Build history of the part. All positions in model axes, mm. A direction names the side the tool comes from. Coordinates: 2 decimals unless noted, no trailing zeros. Order: outer loops, then holes, each group sorted by start corner. A loop starts at its lowest first (then second) coordinate and runs counter-clockwise, first axis right, second up. Notation, with made-up numbers: M 85.5,-26 L 119.5,-26 A10 ccw 119.5,-22 Z; hole C 89.5,-15 d3. An arc over 180 degrees is marked long. Use a Markdown table: item, result. Add a question column.
from build123d import *

# Parameters (mm, degrees)
ESTRUSIONE_ESTRUSIONE1_DEPTH = 2
SCHIZZO2_W                   = 7
SCHIZZO2_H                   = 5
ESTRUSIONE_ESTRUSIONE2_DEPTH = 6.5
FORO_PER_VITE_M3_1_D         = 3.4
FORO_PER_VITE_M3_1_DEPTH     = 2
FORO_PER_VITE_M3_1_TIP       = 1.021463052
FORO_PER_VITE_M3_2_D         = 3.4
RACCORDO1_RADIUS             = 3.5
RACCORDO1_LENGTH             = 5
SMUSSO1_SIZE                 = 1
RACCORDO2_R                  = 1


with BuildPart() as part:
    # Schizzo1 → Estrusione-Estrusione1 (new body)
    with BuildSketch(Plane.XY):
        Polygon((5, 5), (5, 0), (14, 0), (14, -5), (5, -5), (-5, -5), (-5, 5), align=None)
    extrude(amount=ESTRUSIONE_ESTRUSIONE1_DEPTH)

    # Schizzo2 → Estrusione-Estrusione2 (add)
    with BuildSketch(Plane.XY.offset(2)):
        with Locations((10.5, -2.5)):
            Rectangle(SCHIZZO2_W, SCHIZZO2_H)
    extrude(amount=ESTRUSIONE_ESTRUSIONE2_DEPTH)

    # Foro per Vite M3-1
    with Locations(Plane.XY.offset(2)):
        with Locations((0, 0)):
            Hole(FORO_PER_VITE_M3_1_D / 2, depth=FORO_PER_VITE_M3_1_DEPTH)
            with Locations((0, 0, -(FORO_PER_VITE_M3_1_DEPTH + FORO_PER_VITE_M3_1_TIP / 2))):  # 118° drill point
                Cone(0, FORO_PER_VITE_M3_1_D / 2, FORO_PER_VITE_M3_1_TIP, mode=Mode.SUBTRACT)

    # Foro per Vite M3-2 (through all)
    with Locations(Plane(origin=(0, -5, 0), x_dir=(-1, 0, 0), z_dir=(0, -1, 0))):
        with Locations((-10.5, -5.25)):
            Hole(FORO_PER_VITE_M3_2_D / 2)

    # Raccordo1: full round fillet: the end face becomes a half cylinder, R = half its width
    raccordo1_face = Plane((10.5, -2.5, 8.5), x_dir=(0, 1, 0), z_dir=(0, 0, 1))  # on the end face: x along it, z out of the body
    raccordo1_slab = raccordo1_face.offset(-RACCORDO1_RADIUS / 2) * Box(RACCORDO1_LENGTH, 2 * RACCORDO1_RADIUS, RACCORDO1_RADIUS, mode=Mode.PRIVATE)  # the body's end, R deep
    raccordo1_round = Plane((10.5, -2.5, 5), x_dir=(0, 0, 1), z_dir=(0, 1, 0)) * Cylinder(RACCORDO1_RADIUS, RACCORDO1_LENGTH, mode=Mode.PRIVATE)  # its axis R under the face
    add(raccordo1_slab - raccordo1_round, mode=Mode.SUBTRACT)

    # Smusso1
    smusso1_edges = [part.edges().sort_by_distance(p)[0] for p in [
        (14, -2.5, 0),
    ]]
    chamfer(smusso1_edges, length=SMUSSO1_SIZE)

    # Raccordo2
    raccordo2_edges = [part.edges().sort_by_distance(p)[0] for p in [
        (14, -2.5, 1),
        (13, -2.5, 0),
    ]]
    fillet(raccordo2_edges, radius=RACCORDO2_R)


solid = part.part
(1) Drop flat-ended pins along their axis: P1, Ø3, axis at y = 1, z = 7, coming from the -X side; P2, Ø2.5, axis at x = 0, y = 0, coming from the +Z side; P3, Ø4, axis at x = 8, z = 3.5, coming from the +Y side; P4, Ø1, axis at y = 2, z = 1, coming from the +X side. Give the stop position or say it passes through.
(2) Slice it at B-B on x = 10.5. Give the cut face in (y, z).
(3) Drill centre lines: line 1 along Y through (x, z) = (0, 0.5); line 2 along Z through (x, y) = (3.25, -4); line 3 along X through (y, z) = (-1.25, 5.25). Where is each one in solid material? Low to high. Write a range as from..to.
(4) Slice it at D-D on x = 5.25. Give the cut face in (y, z), and give its area (3 significant figures).
(5) Slice it at A-A on y = -2.5. Give the cut face in (x, z).
(6) Which spindle directions (+Z, -Z, +X, -X, +Y, -Y) get a long thin tool onto all of the face, cutting with end or side? Do faces 4 (the cylindrical face through (10.4, -2.5, 8.5)), 5 (the flat face through (1, -2, 2)), 6 (the flat face through (5, 3, 1)). Say none if no direction does.
(7) Slice it at C-C on z = 5.25. Give the cut face in (x, y).
(8) Mould opens along X. For faces 1 (the flat face through (7, -3, 3)), 2 (the flat face through (0, 5, 1)), 3 (the cylindrical face through (0.37, -1.66, 0.99)) say: released by +X, released by -X, zero draft, split by the parting line, or undercut.
Solutions:
| question | item | result |
|---|---|---|
| 1 | P1 | x = 7.11 |
| 1 | P2 | through |
| 1 | P3 | y = 0 |
| 1 | P4 | x = 5 |
| 2 | outline | M -5,0 L 0,0 L 0,3.55 L -5,3.55 Z; M -5,6.95 L 0,6.95 L 0,8.5 L -5,8.5 Z |
| 3 | line 1 | -5..-1.7, 1.7..5 |
| 3 | line 2 | 0..2 |
| 3 | line 3 | 7.01..8.8, 12.2..13.99 |
| 4 | outline | M -5,0 L 0,0 L 0,2 L -5,2 Z |
| 4 | area | 10.0 mm² |
| 5 | outline | M -5,0 L 12.59,0 A1 ccw 13.29,0.29 L 13.71,0.71 A1 ccw 14,1.41 L 14,5 A3.5 ccw 7,5 L 7,2 L -5,2 Z; hole C 10.5,5.25 d3.4 |
| 6 | face 4 | +Z, +Y, -Y |
| 6 | face 5 | +Z, -X, +Y, -Y |
| 6 | face 6 | +Z, -Z, +X, +Y |
| 7 | outline | M 7.01,-5 L 8.8,-5 L 8.8,0 L 7.01,0 Z; M 12.2,-5 L 13.99,-5 L 13.99,0 L 12.2,0 Z |
| 8 | face 1 | released by -X |
| 8 | face 2 | zero draft |
| 8 | face 3 | undercut |
